Drawing for the job (mm, zero at the part's lowest x, y, z). A direction names the side the tool comes from. Give positions to 0.01 mm unless a question says otherwise; leave off trailing zeros. Order: outer loops, then holes, each group sorted by start corner. A loop starts at its lowest first (then second) coordinate and runs counter-clockwise, first axis right, second up. Notation, with made-up numbers: (-16, -20.75) -> (9, -20.75) arc R8 ccw to (9, -11.75) -> close; hole circle Ø11 at (29, 53.25). An arc over 180 degrees is marked (long way). One line per item, written item: value. Start each with the question number.
(1) Saw through at A-A on x = 25.4. Give the cut face in (y, z), plus the area to 4 significant figures.
(2) Two-plate mould, pull along X, no slides. Class the marked faces 1, 2 and 3: +X half, -X half, draft (parallel to the pull), parting line (faces both ways), or undercut.
(3) Probe line 1 (Y direction, x = 25.4, z = 80); line 2 (X direction, y = 17, z = 88) (1 decimal); line 3 (X direction, y = 22.5, z = 89) (1 decimal). List the from-to ranges inside material, lowest first.
(4) Which spindle directions (+Z, -Z, +X, -X, +Y, -Y) get a long thin tool onto all of the face, cutting with end or side? Do the marked faces 4 and 5. Say none if no direction does.
(5) Saw through at C-C on z = 64. Give the cut face in (x, y).
(6) Pin check, flat tips, straight feed: pin 1 (1.5 mm diameter, centred on x = 42.5, z = 79.5, fed in from +Y); pin 2 (3 mm diameter, centred on x = 11, z = 81, fed in from +Y); pin 3 (5 mm diameter, centred on x = 41, y = 9, fed in from -Z); pin 4 (14.5 mm diameter, centred on x = 38.39, y = 17.9, fed in from +Z). Stop position of each tip, or through.
(7) Saw through at D-D on y = 40.4. Give the cut face in (x, z), plus the area to 3 significant figures.
(8) Saw through at B-B on y = 25.4. Give the cut face in (x, z).
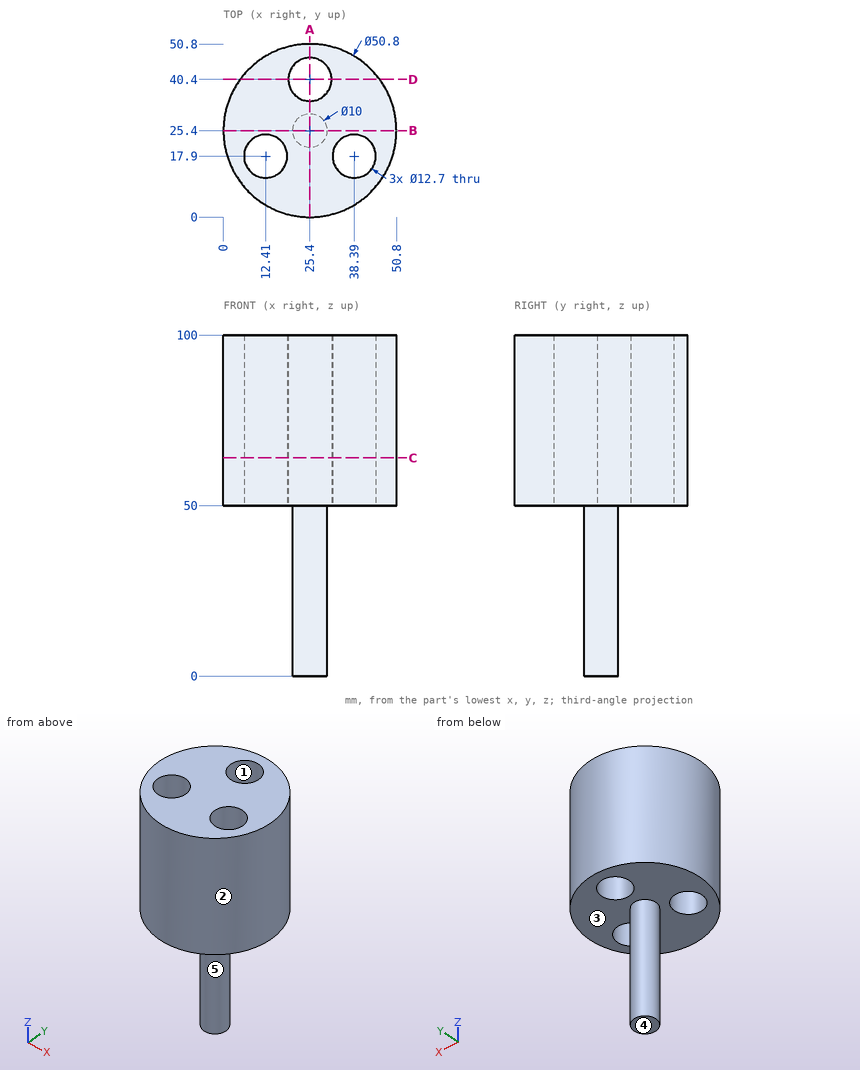
Results below:
1. outline: (0, 50) -> (20.4, 50) -> (20.4, 0) -> (30.4, 0) -> (30.4, 50) -> (34.05, 50) -> (34.05, 100) -> (0, 100) -> close; (46.75, 50) -> (50.8, 50) -> (50.8, 100) -> (46.75, 100) -> close
1. area: 2,405 mm²
2. face 1: undercut
2. face 2: parting line
2. face 3: draft
3. line 1: y = 0 to 34.05, 46.75 to 50.8
3. line 2: x = 1.4 to 6.1, 18.7 to 32.1, 44.7 to 49.4
3. line 3: x = 0.2 to 8, 16.8 to 34, 42.8 to 50.6
4. face 4: -Z, +X, -X, +Y, -Y
4. face 5: -Z
5. outline: circle Ø50.8 at (25.4, 25.4); hole circle Ø12.7 at (12.41, 17.9); hole circle Ø12.7 at (25.4, 40.4); hole circle Ø12.7 at (38.39, 17.9)
6. pin 1: stops at y = 44.84
6. pin 2: stops at y = 47.28
6. pin 3: stops at z = 50
6. pin 4: stops at z = 100
7. outline: (4.9, 50) -> (19.05, 50) -> (19.05, 100) -> (4.9, 100) -> close; (31.75, 50) -> (45.9, 50) -> (45.9, 100) -> (31.75, 100) -> close
7. area: 1,410 mm²
8. outline: (0, 50) -> (20.4, 50) -> (20.4, 0) -> (30.4, 0) -> (30.4, 50) -> (50.8, 50) -> (50.8, 100) -> (0, 100) -> close
